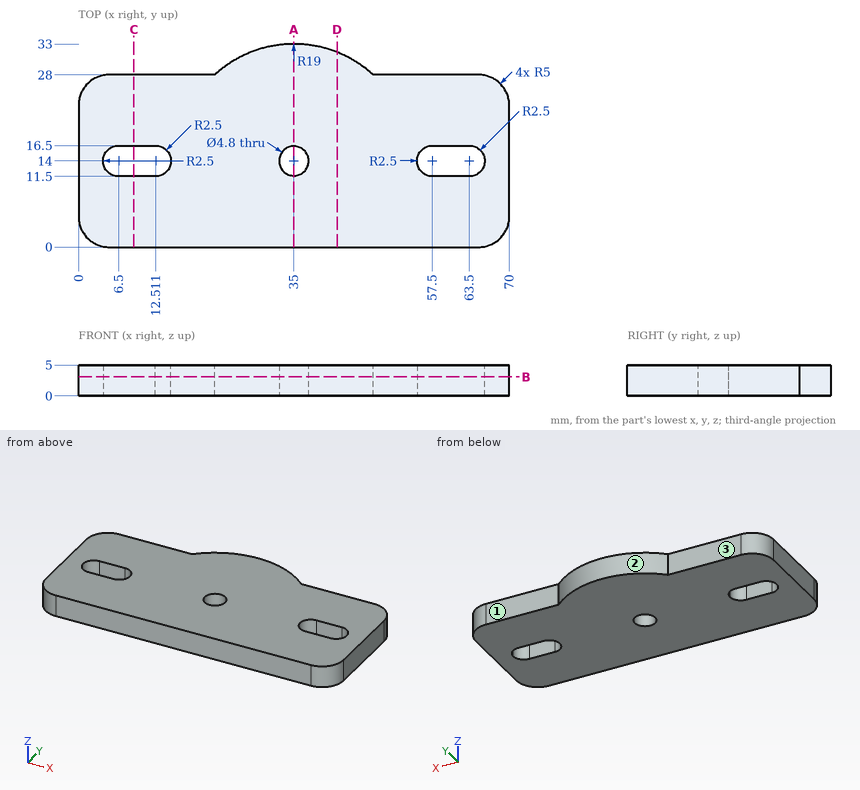
Answer from the drawing. Dimensions are ordinates in mm from the lowest x, y and z of the part. A direction names the side the tool comes from. Give positions to 0.01 mm unless a question says otherwise; leave off trailing zeros. Write each loop counter-clockwise with the first axis right and the second up, starting at its lowest first coordinate (ties: lowest second). Pieces come first, ordered by that corner, then holes. Notation, with made-up numbers: (60.25, 14) -> (86.25, 14) arc R5 cw to (86.25, 21) -> close; hole circle Ø6 at (0, 45.5). An arc over 180 degrees is marked (long way). Use a Markdown table: item, result.
(1) Flat-ended cylindrical pins translate along their axes: P1, Ø2.5, axis at x = 8.5, z = 2, coming from the +Y side; P2, Ø4, axis at x = 35, y = 14, coming from the -Z side. Find the tip coordinate at first contact, or state that the pin passes through.
Return value:
| item | result |
|---|---|
| P1 | y = 28 |
| P2 | through |
(2) Section A-A, the plane x = 35 is taken. Determine the outline of the cut face in (y, z).
Return value:
| item | result |
|---|---|
| outline | (0, 0) -> (11.6, 0) -> (11.6, 5) -> (0, 5) -> close; (16.4, 0) -> (33, 0) -> (33, 5) -> (16.4, 5) -> close |
(3) For the marked faces 1, 2 and 3, determine the directions among +Z, -Z, +X, -X, +Y, -Y from which every point of the face is accessible in a straight line to the end or side of a thin tool.
Return value:
| item | result |
|---|---|
| face 1 | +Z, -Z, +X, +Y |
| face 2 | +Z, -Z, +Y |
| face 3 | +Z, -Z, -X, +Y |
(4) Find the intervals of material crossed by probe 1 along Y at (x, z) = (61.5, 1.4); probe 2 along X at (y, z) = (15, 3.45); probe 3 along X at (y, z) = (16, 4.4) (1 decimal), in increasing order. Write a range as from..to.
Return value:
| item | result |
|---|---|
| probe 1 | 0..11.5, 16.5..28 |
| probe 2 | 0..4.21, 14.8..32.82, 37.18..55.21, 65.79..70 |
| probe 3 | 0..5, 14..33.7, 36.3..56, 65..70 |
(5) Section D-D, the plane x = 42 is taken. Determine the outline of the cut face in (y, z), then the cut area to 3 significant figures.
Return value:
| item | result |
|---|---|
| outline | (0, 0) -> (31.66, 0) -> (31.66, 5) -> (0, 5) -> close |
| area | 158 mm2 |
(6) Section C-C, the plane x = 9 is taken. Determine the outline of the cut face in (y, z), then the cut area to 3 significant figures.
Return value:
| item | result |
|---|---|
| outline | (0, 0) -> (11.5, 0) -> (11.5, 5) -> (0, 5) -> close; (16.5, 0) -> (28, 0) -> (28, 5) -> (16.5, 5) -> close |
| area | 115 mm2 |
(7) Section B-B, the plane z = 3.1 is taken. Determine the outline of the cut face in (x, y) (1 decimal), then the cut area to 3 significant figures.
Return value:
| item | result |
|---|---|
| outline | (0, 5) arc R5 ccw to (5, 0) -> (65, 0) arc R5 ccw to (70, 5) -> (70, 23) arc R5 ccw to (65, 28) -> (47.8, 28) arc R19 ccw to (22.2, 28) -> (5, 28) arc R5 ccw to (0, 23) -> close; hole (6.5, 11.5) -> (12.5, 11.5) arc R2.5 ccw to (15, 14) arc R2.5 ccw to (12.5, 16.5) -> (6.5, 16.5) arc R2.5 ccw to start; hole circle Ø4.8 at (35, 14); hole (57.5, 11.5) -> (63.5, 11.5) arc R2.5 ccw to (63.5, 16.5) -> (57.5, 16.5) arc R2.5 ccw to start |
| area | 1,910 mm2 |
